Source: CAD feature listing. Evaluate the final solid. Frame: model axes, mm. A direction names the side the tool comes from. Coordinates: 2 decimals unless noted, no trailing zeros. Write each loop counter-clockwise with the first axis right and the second up, starting at its lowest first coordinate (ties: lowest second). Pieces come first, ordered by that corner, then holes. Notation, with made-up numbers: (59, 26) - (114, 26) arc R20 ccw to (114, 32) - close; hole circle Ø11 at (19, -2.75). An arc over 180 degrees is marked (long way). One line per item, written item: value.
from build123d import *

# Parameters (mm, degrees)
F3_R     = 1.45
F4_DEPTH = 12


with BuildPart() as f2:
    # F2: sweep along a path in F1
    with BuildLine(Plane.XY) as f2_path:
        Line((-39.078693, 23.98231), (-40, 0))
    # F0 (on Front) → F2 (sweep)
    with BuildSketch(Plane.XZ):
        Polygon((0, 0), (-40, 0), (-40, -12), (7.5, -12), (7.5, -2), (62.5, 6), (87.5, 6), (142.5, -2), (142.5, -12), (190, -12), (190, 0), (150, 0), (150, 9), (0, 9), align=None)
    sweep(path=f2_path.line)

    # F3 (on face) → F4 (cut, through all)
    with BuildSketch(Plane.XY):
        with Locations((178.451802, 11.991155)):
            Circle(F3_R)
        with Locations((-27.530495, 11.991155)):
            Circle(F3_R)
    extrude(amount=-F4_DEPTH, mode=Mode.SUBTRACT)


solid = f2.part
1) Reachability of faces 5 (the flat face through (75, 12, 6)), 6 (the flat face through (-16, 12, -12)), 7 (the flat face through (0.454, 11.823, 4.563)), 8 (the flat face through (150.454, 11.823, 4.437)), 9 (the flat face through (7.954, 11.823, -7.07)) from +Z, -Z, +X, -X, +Y, -Y: full face, straight path, thin tool, end or side. Return the list, or none.
Values found:
face 5: -Z, +Y, -Y
face 6: -Z, +X, -X, +Y, -Y
face 7: +Z, -X, +Y
face 8: +Z, +X, -Y
face 9: -Z, -Y
2) Section query B-B on y = 5.5. Output: boundary loops of the cut face in (x, z), then the cut area to 3 significant figures.
Values found:
outline: (-39.79, -12) - (7.71, -12) - (7.71, -2) - (62.71, 6) - (87.71, 6) - (142.71, -2) - (142.71, -12) - (190.21, -12) - (190.21, 0) - (150.21, 0) - (150.21, 9) - (0.21, 9) - (0.21, 0) - (-39.79, 0) - close
area: 2,120 mm2
3) Contact query for flat-ended pins moving along their axis: P1, Ø4, axis at y = 3.5, z = -4.5, coming from the -X side; P2, Ø7, axis at x = 73, y = 8, coming from the -Z side; P3, Ø2, axis at y = 18.5, z = -1.5, coming from the -X side. Output: stop coordinate, or through.
Values found:
P1: x = -39.94
P2: z = 6
P3: x = -39.33
4) Draft query along X for faces 1 (the flat face through (-39.546, 11.823, -5.916)), 2 (the flat face through (166, 12, -12)), 3 (the flat face through (190.454, 11.823, -6.084)), 4 (the flat face through (142.954, 11.823, -6.93)). Return one class per face: released by +X, released by -X, zero draft, split by the parting line, or undercut.
Values found:
face 1: released by -X
face 2: zero draft
face 3: released by +X
face 4: undercut
5) Section query D-D on x = 45. Output: boundary loops of the cut face in (y, z).
Values found:
outline: (0, 3.45) - (23.98, 3.32) - (23.98, 9) - (0, 9) - close
6) Section query A-A on z = -6.5. Output: boundary loops of the cut face in (x, y), then the cut area to 3 significant figures.
Values found:
outline: (-40, 0) - (7.5, 0) - (8.42, 23.98) - (-39.08, 23.98) - close; (142.5, 0) - (190, 0) - (190.92, 23.98) - (143.42, 23.98) - close; hole circle Ø2.9 at (-27.53, 11.99); hole circle Ø2.9 at (178.45, 11.99)
area: 2,270 mm2
7) Section query C-C on x = -5. Output: boundary loops of the cut face in (y, z).
Values found:
outline: (0, -12) - (23.98, -12) - (23.98, 0) - (0, 0) - close
8) Material intervals for line 1 (Z direction, x = -27, y = 7.25); line 2 (Z direction, x = 72.5, y = 6.75); line 3 (X direction, y = 22.5, z = -6.5), sorted ascending.
Values found:
line 1: -12 to 0
line 2: 6 to 9
line 3: -39.14 to 8.36, 143.36 to 190.86
